Design review of the part built by this model. Coordinates are the model's own, in mm. A direction names the side the tool comes from. Round coordinates to 2 decimals unless told otherwise and drop trailing zeros. Write each loop counter-clockwise with the first axis right and the second up, starting at its lowest first coordinate (ties: lowest second). Pieces come first, ordered by that corner, then holes. Notation, with made-up numbers: (-8, -9.75) -> (30, -9.75) arc R19 ccw to (30, -5.75) -> close; hole circle Ø1 at (36, 56.25). An arc over 180 degrees is marked (long way). One line per question, with ' | ' between items. Start each with the question number.
1) For faces 4 (the flat face through (-3, 2, 0)), 5 (the flat face through (0, 6.5, 0)), list the 3-axis set-ups (+Z, -Z, +X, -X, +Y, -Y) from which the entire face can be reached by the end or side of a thin tool; tool diameter is ignored.
2) Consider section C-C (y = 1.5). Give the boundary of the cut face in (x, z), then the cut area to 3 significant figures.
3) Consider section B-B (y = 3.5). Give the boundary of the cut face in (x, z).
4) For probe 1 along Y at (x, z) = (-1.5, 2.5); probe 2 along Y at (x, z) = (-1.5, -5.25); probe 3 along X at (y, z) = (1, -4), list the stretches that pass through material, from the lowest coordinate up.
5) Consider section A-A (z = 0). Give the boundary of the cut face in (x, y).
6) Mouldability with a two-part tool opening along Y and no side actions: class faces 1 (the flat face through (0, 0, 0)), 2 (the cylindrical face through (-2.44, 3.23, -0.54)), 3 (the cylindrical face through (-4.88, 5.49, -1.08)) as +Y half, -Y half, draft (parallel to the pull), parting line (faces both ways), or undercut.
```python
from build123d import *

# Parameters (mm, degrees)
SKETCH1_R           = 7.5
BOSS_EXTRUDE1_DEPTH = 2
SKETCH2_R           = 2.5
BOSS_EXTRUDE2_DEPTH = 2.5
SKETCH3_R           = 5
BOSS_EXTRUDE3_DEPTH = 2
FILLET1_R           = 0.2


with BuildPart() as part:
    # Sketch1 → Boss-Extrude1 (new body)
    with BuildSketch(Plane(origin=(0, 0, 0), x_dir=(1, 0, 0), z_dir=(0, 1, 0))):
        with Locations(Location((0, 0, 0), (0, 0, 270))):
            Circle(SKETCH1_R)
    extrude(amount=BOSS_EXTRUDE1_DEPTH)

    # Sketch2 → Boss-Extrude2 (add)
    with BuildSketch(Plane(origin=(0, 2, 0), x_dir=(1, 0, 0), z_dir=(0, 1, 0))):
        with Locations(Location((0, 0, 0), (0, 0, 270))):
            Circle(SKETCH2_R)
    extrude(amount=BOSS_EXTRUDE2_DEPTH)

    # Sketch3 → Boss-Extrude3 (add)
    with BuildSketch(Plane(origin=(0, 4.5, 0), x_dir=(1, 0, 0), z_dir=(0, 1, 0))):
        with Locations(Location((0, 0, 0), (0, 0, 270))):
            Circle(SKETCH3_R)
    extrude(amount=BOSS_EXTRUDE3_DEPTH)

    # Fillet1
    fillet1_edges = [part.edges().sort_by_distance(p)[0] for p in [
        (0, 6.5, -5),
        (0, 0, -7.5),
        (0, 2, -7.5),
        (0, 4.5, -5),
    ]]
    fillet(fillet1_edges, radius=FILLET1_R)


solid = part.part
```
From the geometry:
1) face 4: none | face 5: +Z, -Z, +X, -X, +Y
2) outline: circle Ø15 at (0, 0) | area: 177 mm2
3) outline: circle Ø5 at (0, 0)
4) probe 1: y = 0 to 2, 4.5 to 6.5 | probe 2: y = 0 to 2 | probe 3: x = -6.34 to 6.34
5) outline: (-7.5, 0.2) arc R0.2 ccw to (-7.3, 0) -> (7.3, 0) arc R0.2 ccw to (7.5, 0.2) -> (7.5, 1.8) arc R0.2 ccw to (7.3, 2) -> (2.5, 2) -> (2.5, 4.5) -> (4.8, 4.5) arc R0.2 ccw to (5, 4.7) -> (5, 6.3) arc R0.2 ccw to (4.8, 6.5) -> (-4.8, 6.5) arc R0.2 ccw to (-5, 6.3) -> (-5, 4.7) arc R0.2 ccw to (-4.8, 4.5) -> (-2.5, 4.5) -> (-2.5, 2) -> (-7.3, 2) arc R0.2 ccw to (-7.5, 1.8) -> close
6) face 1: -Y half | face 2: undercut | face 3: draft
